Print and shaded views of the part. All mm, measured from the part's lowest x, y and z. A direction names the side the tool comes from. Coordinates: 2 decimals unless noted, no trailing zeros. Order: outer loops, then holes, each group sorted by start corner. A loop starts at its lowest first (then second) coordinate and runs counter-clockwise, first axis right, second up. Notation, with made-up numbers: (-16, 3) - (41, 3) arc R19 cw to (41, 12) - close; hole circle Ø6 at (23, 7). An arc over 180 degrees is marked (long way). Write each question's results on one line, items separated by ' | '.
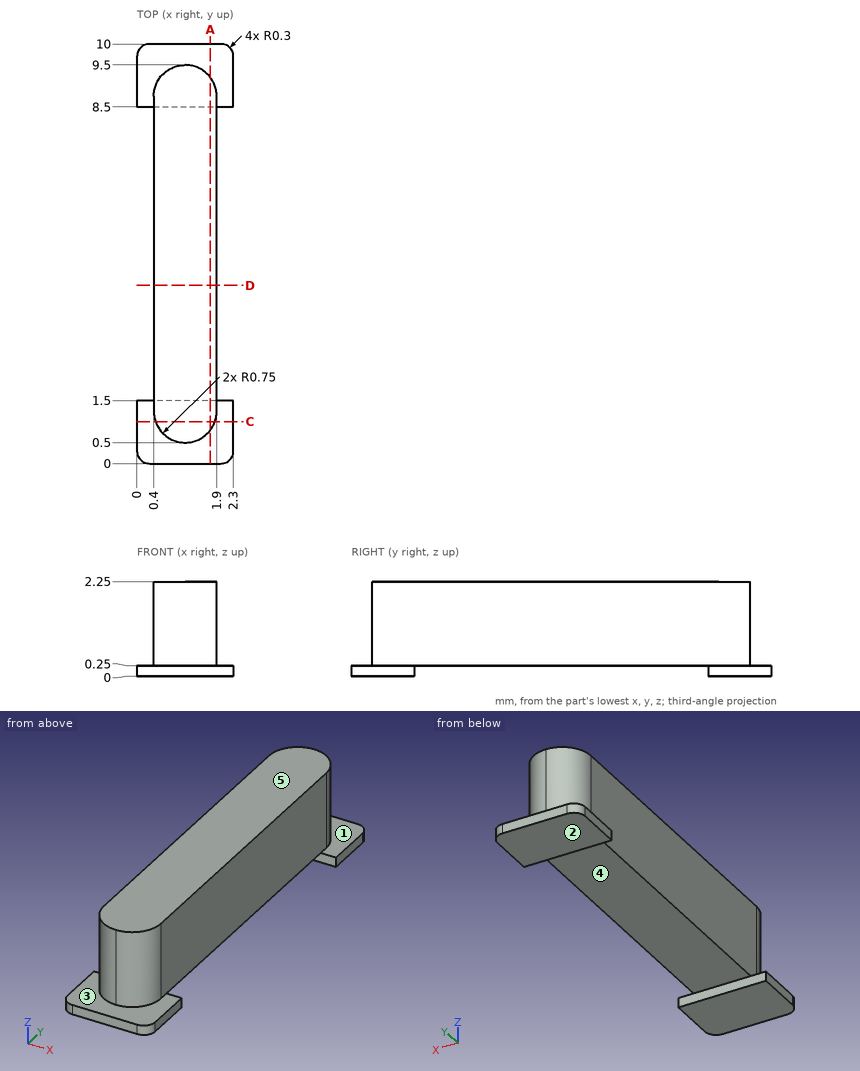
1. Two-plate mould, pull along Y, no slides. Class the marked faces 4 and 5: +Y half, -Y half, draft (parallel to the pull), parting line (faces both ways), or undercut.
Solved:
face 4: undercut | face 5: draft
2. Band-saw the part on A-A on x = 1.75. Give the cut face in (y, z), then the cut area to 4 significant figures.
Solved:
outline: (0, 0) - (1.5, 0) - (1.5, 0.25) - (8.5, 0.25) - (8.5, 0) - (10, 0) - (10, 0.25) - (9.2, 0.25) - (9.2, 2.25) - (0.8, 2.25) - (0.8, 0.25) - (0, 0.25) - close | area: 17.55 mm2
3. Band-saw the part on D-D on y = 4.25. Give the cut face in (x, z).
Solved:
outline: (0.4, 0.25) - (1.9, 0.25) - (1.9, 2.25) - (0.4, 2.25) - close
4. Drop a flat-ended pin along its axis: pin 1 Ø1.2 at (x, y) = (1.5, 5) entering from -Z. Give the stop position or say it passes through.
Solved:
pin 1: stops at z = 0.25
5. Probe line 1 (Z direction, x = 1.6, y = 4.5); line 2 (X direction, y = 8.5, z = 0.45); line 3 (Y direction, x = 1.1, z = 0.95). List the from-to ranges inside material, lowest first.
Solved:
line 1: z = 0.25 to 2.25 | line 2: x = 0.4 to 1.9 | line 3: y = 0.5 to 9.5
6. Band-saw the part on C-C on y = 1. Give the cut face in (x, z), then the cut area to 3 significant figures.
Solved:
outline: (0, 0) - (2.3, 0) - (2.3, 0.25) - (1.86, 0.25) - (1.86, 2.25) - (0.44, 2.25) - (0.44, 0.25) - (0, 0.25) - close | area: 3.40 mm2
7. Tool access for the marked faces 1, 2 and 3: list every direction of +Z, -Z, +X, -X, +Y, -Y with a clear straight run to the whole face (end or side of a thin tool).
Solved:
face 1: +Z, +X, +Y | face 2: -Z, +X, -X, +Y, -Y | face 3: +Z, -X, -Y
